```python
from build123d import *

# Parameters (mm, degrees)
SKETCH1_R           = 4.75
BOSS_EXTRUDE1_DEPTH = 4
SKETCH2_R           = 4
SKETCH2_R_2         = 3.05
BOSS_EXTRUDE2_DEPTH = 6
CHAMFER1_SIZE       = 0.5


with BuildPart() as part:
    # Sketch1 → Boss-Extrude1 (new body)
    with BuildSketch(Plane(origin=(0, 0, 0), x_dir=(1, 0, 0), z_dir=(0, 1, 0))):
        with Locations(Location((0, 0, 0), (0, 0, 270))):
            Circle(SKETCH1_R)
    extrude(amount=BOSS_EXTRUDE1_DEPTH)

    # Sketch2 → Boss-Extrude2 (add)
    with BuildSketch(Plane(origin=(0, 4, 0), x_dir=(1, 0, 0), z_dir=(0, 1, 0))):
        with Locations(Location((0, 0, 0), (0, 0, 270))):
            Circle(SKETCH2_R)
        with Locations(Location((0, 0, 0), (0, 0, 270))):
            Circle(SKETCH2_R_2, mode=Mode.SUBTRACT)
    extrude(amount=BOSS_EXTRUDE2_DEPTH)

    # Chamfer1
    chamfer1_edges = [part.edges().sort_by_distance(p)[0] for p in [
        (0, 0, -4.75),
        (0, 10, -4),
    ]]
    chamfer(chamfer1_edges, length=CHAMFER1_SIZE)


solid = part.part
```
The model under review builds one solid part; all positions refer to its coordinate system, in mm. A direction names the side the tool comes from. Give positions to 0.01 mm unless a question says otherwise; leave off trailing zeros. Write each loop counter-clockwise with the first axis right and the second up, starting at its lowest first coordinate (ties: lowest second). Pieces come first, ordered by that corner, then holes.
(1) To check wall thickness, follow L1, parallel to X at y = 6.2, z = 0; L2, parallel to X at y = 8.25, z = -2.25; L3, parallel to Y at x = 0.75, z = -2. State the ranges of each line that lie inside material, in increasing order.
(2) Consider section B-B, the plane x = 0. Give the boundary of the cut face in (y, z).
(3) Consider section C-C, the plane y = 9. Give the boundary of the cut face in (x, z), and give its area (3 significant figures).
(4) For P1, Ø2, axis at x = -2, y = 3, coming from the -Z side; P2, Ø1.5, axis at y = 8, z = 0.5, coming from the -X side; P3, Ø4, axis at x = -2.5, y = 8, coming from the +Z side, all flat-tipped, find the tip position at first contact; note any pin that passes through.
(5) The part is to be moulded in two halves that separate along X. For faces 1 (the cylindrical face through (-1.856, 6.958, -2.42)), 2 (the flat face through (0, 4, 0)), 3 (the flat face through (0, 0, 0)), 4 (the cylindrical face through (-3.905, 6.712, -0.867)), say which applies: released by +X, released by -X, zero draft, split by the parting line, or undercut.
(6) Tool access review of faces 5 (the flat face through (-2, 4, -4)), 6 (the cylindrical face through (-2.89, 2.23, -3.77)): name each direction out of +Z, -Z, +X, -X, +Y, -Y from which nothing blocks a thin tool from reaching the whole face with its end or side.
(7) Consider section A-A, the plane z = 0. Give the boundary of the cut face in (x, y), and give its area (3 significant figures).
Returned:
1. L1: x = -4 to -3.05, 3.05 to 4
1. L2: x = -3.31 to -2.06, 2.06 to 3.31
1. L3: y = 0 to 4
2. outline: (0, -4.25) - (0.5, -4.75) - (4, -4.75) - (4, -4) - (9.5, -4) - (10, -3.5) - (10, -3.05) - (4, -3.05) - (4, 3.05) - (10, 3.05) - (10, 3.5) - (9.5, 4) - (4, 4) - (4, 4.75) - (0.5, 4.75) - (0, 4.25) - close
3. outline: circle Ø8 at (0, 0); hole circle Ø6.1 at (0, 0)
3. area: 21.0 mm2
4. P1: stops at z = -4.64
4. P2: stops at x = -4
4. P3: stops at z = 3.97
5. face 1: undercut
5. face 2: undercut
5. face 3: zero draft
5. face 4: split by the parting line
6. face 5: +Y
6. face 6: +Y, -Y
7. outline: (-4.75, 0.5) - (-4.25, 0) - (4.25, 0) - (4.75, 0.5) - (4.75, 4) - (4, 4) - (4, 9.5) - (3.5, 10) - (3.05, 10) - (3.05, 4) - (-3.05, 4) - (-3.05, 10) - (-3.5, 10) - (-4, 9.5) - (-4, 4) - (-4.75, 4) - close
7. area: 48.9 mm2
